Source: CAD feature listing. Evaluate the final solid. Frame: model axes, mm. Face numbers are marked on the shaded views. A direction names the side the tool comes from. Round coordinates to 2 decimals unless told otherwise and drop trailing zeros. Order: outer loops, then holes, each group sorted by start corner. A loop starts at its lowest first (then second) coordinate and runs counter-clockwise, first axis right, second up. Notation, with made-up numbers: M 36,69.5 L 52,69.5 A11 ccw 52,81.5 Z; hole C 80,-30.5 d11. An arc over 180 degrees is marked long. Answer in a Markdown table with one row per item. Add a question column.
Autodesk Inventor part; units mm, degrees
ref_plane "YZ Plane" through (0, 0, 0) normal (1, 0, 0) x (0, 1, 0)
ref_plane "XZ Plane" through (0, 0, 0) normal (0, 1, 0) x (-1, 0, 0)
ref_plane "XY Plane" through (0, 0, 0) normal (0, 0, 1) x (1, 0, 0)
sketch "Sketch1" plane through (0, 0, 0) normal (0, 0, 1) x (1, 0, 0)
  circle A0 centre (0, 0) radius 10.3
  circle A1 centre (0, 0) radius 1.45
  dimension "d0" = 20.6
  dimension "d7" = 2.9
extrude "Extrusion1" add sketch "Sketch1" along normal blind 2.2
sketch "Sketch2" plane through (0, 0, 2.2) normal (0, 0, 1) x (1, 0, 0)
  circle A0 centre (0, 0) radius 4.4
  circle A1 centre (0, 0) radius 2.5
  dimension "d3" = 8.8
  dimension "d4" = 5
extrude "Extrusion2" add sketch "Sketch2" along normal blind 3.3
properties part number "orczyk serwa okrągły 02-2"
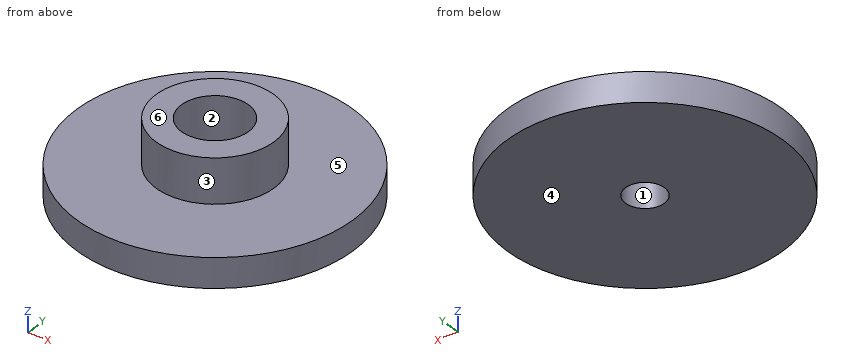
(1) Cut plane C-C (z = 0.55). Return loops of the section in (x, y).
(2) Cut plane A-A (y = 0). Return loops of the section in (x, z), and give its area (3 significant figures).
(3) Pin query (flat end, axial travel): pin 1 (3 mm diameter, centred on x = 6.5, y = 1, fed in from +Z); pin 2 (6.5 mm diameter, centred on x = 0, y = 0, fed in from +Z); pin 3 (1.5 mm diameter, centred on y = 5.5, z = 2.5, fed in from -X); pin 4 (1.5 mm diameter, centred on y = 6.5, z = 2.5, fed in from -X). Return the tip coordinate at first contact, or that it passes through.
(4) Access query for the marked faces 5 and 6. Directions: +Z, -Z, +X, -X, +Y, -Y. A direction counts if a zero-diameter tool reaches every point of the face in a straight line with its end or side. Return the directions, or none.
(5) Line query: line 1 (Y direction, x = 0, z = 1.25); line 2 (Y direction, x = 0, z = 4.35); line 3 (Z direction, x = 3.5, y = 4.5). Output: solid intervals per line, ascending. Write a range as from..to.
(6) Cut plane D-D (z = 4.4). Return loops of the section in (x, y).
(7) Draft query along Y for the marked faces 1, 2, 3 and 4. Return one class per face: +Y half, -Y half, draft (parallel to the pull), parting line (faces both ways), or undercut.
Answer list:
| question | item | result |
|---|---|---|
| 1 | outline | C 0,0 d20.6; hole C 0,0 d2.9 |
| 2 | outline | M -10.3,0 L -1.45,0 L -1.45,2.2 L -2.5,2.2 L -2.5,5.5 L -4.4,5.5 L -4.4,2.2 L -10.3,2.2 Z; M 1.45,0 L 10.3,0 L 10.3,2.2 L 4.4,2.2 L 4.4,5.5 L 2.5,5.5 L 2.5,2.2 L 1.45,2.2 Z |
| 2 | area | 51.5 mm² |
| 3 | pin 1 | z = 2.2 |
| 3 | pin 2 | z = 5.5 |
| 3 | pin 3 | x = -9.11 |
| 3 | pin 4 | x = -8.5 |
| 4 | face 5 | +Z |
| 4 | face 6 | +Z, +X, -X, +Y, -Y |
| 5 | line 1 | -10.3..-1.45, 1.45..10.3 |
| 5 | line 2 | -4.4..-2.5, 2.5..4.4 |
| 5 | line 3 | 0..2.2 |
| 6 | outline | C 0,0 d8.8; hole C 0,0 d5 |
| 7 | face 1 | undercut |
| 7 | face 2 | undercut |
| 7 | face 3 | parting line |
| 7 | face 4 | draft |
